Can you work these out from the model? Positions are in its coordinate system, mm. Face numbers are marked on the shaded views. A direction names the side the tool comes from. Give positions to 0.01 mm unless a question says otherwise; leave off trailing zeros. Write each loop counter-clockwise with the first axis right and the second up, starting at its lowest first coordinate (ties: lowest second). Pieces come first, ordered by that corner, then holes.
1. Suppose I cut it at A-A (y = 28). Please give me the cut outline in (x, z) (1 decimal).
2. Suppose I cut it at B-B (y = 21). Please give me the cut outline in (x, z) (3 decimals), and give its area (3 significant figures).
3. On a 3-axis mill with a long thin cutter (end or side, diameter ignored), from which of +Z, -Z, +X, -X, +Y, -Y can I reach the whole of each face in a straight line? I mean the marked faces 1 and 2. Say none if no direction works.
4. I'm going to push flat-ended pins straight in: pin 1 (2.5 mm diameter, centred on x = 74.61, z = 4.76, fed in from -Y); pin 2 (3 mm diameter, centred on x = 4.76, z = 74.61, fed in from +Y); pin 3 (2.5 mm diameter, centred on x = 4.76, z = 74.61, fed in from +Y). Where does each tip first touch, or does it pass through?
5. Suppose I cut it at C-C (x = 56). Please give me the cut outline in (y, z) (3 decimals).
6. If I drill on probe 1 along X at (y, z) = (20.5, 93) (3 decimals); probe 2 along Z at (x, y) = (75, 6) (3 decimals), over which ranges is the centre line in solid material (lowest first)?
7. Suppose I cut it at D-D (z = 98.5). Please give me the cut outline in (x, y) (3 decimals).
```python
from build123d import *

# Parameters (mm, degrees)
BOSS_EXTRUDE1_DEPTH                           = 38.1
CBORE_FOR_4_SOCKET_HEAD_CAP_SCREW1_AT_2_COUNT = 2
CBORE_FOR_4_SOCKET_HEAD_CAP_SCREW1_AT_2_PITCH = 34.925
CBORE_FOR_4_SOCKET_HEAD_CAP_SCREW1_AT_3_COUNT = 2
CBORE_FOR_4_SOCKET_HEAD_CAP_SCREW1_AT_3_PITCH = 69.85
CBORE_FOR_4_SOCKET_HEAD_CAP_SCREW1_AT_4_COUNT = 2
CBORE_FOR_4_SOCKET_HEAD_CAP_SCREW1_AT_4_PITCH = 34.925
CBORE_FOR_4_SOCKET_HEAD_CAP_SCREW1_AT_5_COUNT = 2
CBORE_FOR_4_SOCKET_HEAD_CAP_SCREW1_AT_5_PITCH = 69.85
CBORE_FOR_4_SOCKET_HEAD_CAP_SCREW1_AT_6_COUNT = 2
CBORE_FOR_4_SOCKET_HEAD_CAP_SCREW1_AT_6_PITCH = 104.775
CHAMFER1_SIZE                                 = 0.508


with BuildPart() as part:
    # Sketch1 → Boss-Extrude1 (new body)
    with BuildSketch(Plane(origin=(0, 0, 0), x_dir=(1, 0, 0), z_dir=(0, 1, 0))):
        Polygon((0, 0), (85.725, 0), (85.725, -9.525), (9.525, -9.525), (9.525, -123.825), (0, -123.825), align=None)
    extrude(amount=BOSS_EXTRUDE1_DEPTH)

    # Sketch2 → CBORE for #4 Socket Head Cap Screw1 (revolve, cut)
    with BuildSketch(Plane(origin=(4.7625, 0, 4.7625), x_dir=(0, 0, -1), z_dir=(1, 0, 0))):
        Polygon((0, 0), (0, 13.680574487), (1.63195, 12.7), (1.63195, 4.7625), (1.984375, 4.7625), (1.984375, 0), align=None)
    cbore_for_4_socket_head_cap_screw1 = revolve(axis=Axis((4.7625, -6.35, 4.7625), (0, 1, 0)), mode=Mode.SUBTRACT)

    # CBORE for #4 Socket Head Cap Screw1 at 2: CBORE for #4 Socket Head Cap Screw1 ×2
    with Locations(*[(0, 0, i * CBORE_FOR_4_SOCKET_HEAD_CAP_SCREW1_AT_2_PITCH) for i in range(1, CBORE_FOR_4_SOCKET_HEAD_CAP_SCREW1_AT_2_COUNT)]):
        add(cbore_for_4_socket_head_cap_screw1, mode=Mode.SUBTRACT)

    # CBORE for #4 Socket Head Cap Screw1 at 3: CBORE for #4 Socket Head Cap Screw1 ×2
    with Locations(*[(0, 0, i * CBORE_FOR_4_SOCKET_HEAD_CAP_SCREW1_AT_3_PITCH) for i in range(1, CBORE_FOR_4_SOCKET_HEAD_CAP_SCREW1_AT_3_COUNT)]):
        add(cbore_for_4_socket_head_cap_screw1, mode=Mode.SUBTRACT)

    # CBORE for #4 Socket Head Cap Screw1 at 4: CBORE for #4 Socket Head Cap Screw1 ×2
    with Locations(*[(i * CBORE_FOR_4_SOCKET_HEAD_CAP_SCREW1_AT_4_PITCH, 0, 0) for i in range(1, CBORE_FOR_4_SOCKET_HEAD_CAP_SCREW1_AT_4_COUNT)]):
        add(cbore_for_4_socket_head_cap_screw1, mode=Mode.SUBTRACT)

    # CBORE for #4 Socket Head Cap Screw1 at 5: CBORE for #4 Socket Head Cap Screw1 ×2
    with Locations(*[(i * CBORE_FOR_4_SOCKET_HEAD_CAP_SCREW1_AT_5_PITCH, 0, 0) for i in range(1, CBORE_FOR_4_SOCKET_HEAD_CAP_SCREW1_AT_5_COUNT)]):
        add(cbore_for_4_socket_head_cap_screw1, mode=Mode.SUBTRACT)

    # CBORE for #4 Socket Head Cap Screw1 at 6: CBORE for #4 Socket Head Cap Screw1 ×2
    with Locations(*[(0, 0, i * CBORE_FOR_4_SOCKET_HEAD_CAP_SCREW1_AT_6_PITCH) for i in range(1, CBORE_FOR_4_SOCKET_HEAD_CAP_SCREW1_AT_6_COUNT)]):
        add(cbore_for_4_socket_head_cap_screw1, mode=Mode.SUBTRACT)

    # Mirror CBORE for #4 Socket Head Cap Screw: CBORE for #4 Socket Head Cap Screw1 across plane
    add(cbore_for_4_socket_head_cap_screw1.mirror(Plane.ZX.offset(19.05)), mode=Mode.SUBTRACT)

    # Mirror CBORE for _4 Socket Head Cap  2 → Mirror CBORE for _4 Socket Head Cap  3 (revolve, cut)
    with BuildSketch(Plane(origin=(4.7625, 38.1, 39.6875), x_dir=(0, 0, -1), z_dir=(1, 0, 0))):
        Polygon((0, 0), (0, -13.680574487), (1.63195, -12.7), (1.63195, -4.7625), (1.984375, -4.7625), (1.984375, 0), align=None)
    revolve(axis=Axis((4.7625, 44.45, 39.6875), (0, 1, 0)), mode=Mode.SUBTRACT)

    # Mirror CBORE for _4 Socket Head Cap  4 → Mirror CBORE for _4 Socket Head Cap  5 (revolve, cut)
    with BuildSketch(Plane(origin=(4.7625, 38.1, 74.6125), x_dir=(0, 0, -1), z_dir=(1, 0, 0))):
        Polygon((0, 0), (0, -13.680574487), (1.63195, -12.7), (1.63195, -4.7625), (1.984375, -4.7625), (1.984375, 0), align=None)
    revolve(axis=Axis((4.7625, 44.45, 74.6125), (0, 1, 0)), mode=Mode.SUBTRACT)

    # Mirror CBORE for _4 Socket Head Cap  6 → Mirror CBORE for _4 Socket Head Cap  7 (revolve, cut)
    with BuildSketch(Plane(origin=(39.6875, 38.1, 4.7625), x_dir=(0, 0, -1), z_dir=(1, 0, 0))):
        Polygon((0, 0), (0, -13.680574487), (1.63195, -12.7), (1.63195, -4.7625), (1.984375, -4.7625), (1.984375, 0), align=None)
    revolve(axis=Axis((39.6875, 44.45, 4.7625), (0, 1, 0)), mode=Mode.SUBTRACT)

    # Mirror CBORE for _4 Socket Head Cap  8 → Mirror CBORE for _4 Socket Head Cap  9 (revolve, cut)
    with BuildSketch(Plane(origin=(74.6125, 38.1, 4.7625), x_dir=(0, 0, -1), z_dir=(1, 0, 0))):
        Polygon((0, 0), (0, -13.680574487), (1.63195, -12.7), (1.63195, -4.7625), (1.984375, -4.7625), (1.984375, 0), align=None)
    revolve(axis=Axis((74.6125, 44.45, 4.7625), (0, 1, 0)), mode=Mode.SUBTRACT)

    # Mirror CBORE for _4 Socket Head Cap  10 → Mirror CBORE for _4 Socket Head Cap  11 (revolve, cut)
    with BuildSketch(Plane(origin=(4.7625, 38.1, 109.5375), x_dir=(0, 0, -1), z_dir=(1, 0, 0))):
        Polygon((0, 0), (0, -13.680574487), (1.63195, -12.7), (1.63195, -4.7625), (1.984375, -4.7625), (1.984375, 0), align=None)
    revolve(axis=Axis((4.7625, 44.45, 109.5375), (0, 1, 0)), mode=Mode.SUBTRACT)

    # Chamfer1
    # the kernel refuses this chamfer: 0.508 mm, written as the material it adds along each edge
    with BuildSketch(Plane(origin=(4.7625, 4.7625, 4.7625), x_dir=(0, 0, -1), z_dir=(1, 0, 0))) as chamfer1_piece_1_section:
        Polygon((1.984375, -CHAMFER1_SIZE), (1.984375 - CHAMFER1_SIZE, 0), (1.984375, 0), align=None)
    chamfer1_piece_1 = revolve(axis=Axis((4.7625, 4.7625, 4.7625), (0, 1, 0)), mode=Mode.PRIVATE)
    chamfer1_piece_1 = chamfer1_piece_1 - Plane(origin=(4.7625, 4.431570678, 4.7625), x_dir=(0, 0, -1), z_dir=(0, -1, 0)) * Cylinder(1.63195, 8, mode=Mode.PRIVATE)
    add(chamfer1_piece_1)
    with BuildSketch(Plane(origin=(4.7625, 4.7625, 74.6125), x_dir=(0, 0, -1), z_dir=(1, 0, 0))) as chamfer1_piece_2_section:
        Polygon((1.984375, -CHAMFER1_SIZE), (1.984375 - CHAMFER1_SIZE, 0), (1.984375, 0), align=None)
    chamfer1_piece_2 = revolve(axis=Axis((4.7625, 4.7625, 74.6125), (0, 1, 0)), mode=Mode.PRIVATE)
    chamfer1_piece_2 = chamfer1_piece_2 - Plane(origin=(4.7625, 4.431570678, 74.6125), x_dir=(0, 0, -1), z_dir=(0, -1, 0)) * Cylinder(1.63195, 8, mode=Mode.PRIVATE)
    add(chamfer1_piece_2)
    with BuildSketch(Plane(origin=(39.6875, 33.3375, 4.7625), x_dir=(0, 0, -1), z_dir=(1, 0, 0))) as chamfer1_piece_3_section:
        Polygon((1.984375, CHAMFER1_SIZE), (1.984375 - CHAMFER1_SIZE, 0), (1.984375, 0), align=None)
    chamfer1_piece_3 = revolve(axis=Axis((39.6875, 33.3375, 4.7625), (0, 1, 0)), mode=Mode.PRIVATE)
    chamfer1_piece_3 = chamfer1_piece_3 - Plane(origin=(39.6875, 33.668429322, 4.7625), x_dir=(0, 0, -1), z_dir=(0, 1, 0)) * Cylinder(1.63195, 8, mode=Mode.PRIVATE)
    add(chamfer1_piece_3)
    # the kernel refuses this chamfer: 0.508 mm, written as the material it takes off along each edge
    with BuildSketch(Plane(origin=(4.7625, 0, 4.7625), x_dir=(0, 0, -1), z_dir=(1, 0, 0))) as chamfer1_2_piece_1:
        Polygon((1.984375 + CHAMFER1_SIZE, 0), (1.984375, CHAMFER1_SIZE), (1.984375, 0), align=None)
    revolve(axis=Axis((4.7625, 0, 4.7625), (0, 1, 0)), mode=Mode.SUBTRACT)
    with BuildSketch(Plane(origin=(4.7625, 0, 74.6125), x_dir=(0, 0, -1), z_dir=(1, 0, 0))) as chamfer1_2_piece_2:
        Polygon((1.984375 + CHAMFER1_SIZE, 0), (1.984375, CHAMFER1_SIZE), (1.984375, 0), align=None)
    revolve(axis=Axis((4.7625, 0, 74.6125), (0, 1, 0)), mode=Mode.SUBTRACT)
    with BuildSketch(Plane(origin=(74.6125, 0, 4.7625), x_dir=(0, 0, -1), z_dir=(1, 0, 0))) as chamfer1_2_piece_3:
        Polygon((1.984375 + CHAMFER1_SIZE, 0), (1.984375, CHAMFER1_SIZE), (1.984375, 0), align=None)
    revolve(axis=Axis((74.6125, 0, 4.7625), (0, 1, 0)), mode=Mode.SUBTRACT)
    with BuildSketch(Plane(origin=(39.6875, 0, 4.7625), x_dir=(0, 0, -1), z_dir=(1, 0, 0))) as chamfer1_2_piece_4:
        Polygon((1.984375 + CHAMFER1_SIZE, 0), (1.984375, CHAMFER1_SIZE), (1.984375, 0), align=None)
    revolve(axis=Axis((39.6875, 0, 4.7625), (0, 1, 0)), mode=Mode.SUBTRACT)
    with BuildSketch(Plane(origin=(4.7625, 0, 39.6875), x_dir=(0, 0, -1), z_dir=(1, 0, 0))) as chamfer1_2_piece_5:
        Polygon((1.984375 + CHAMFER1_SIZE, 0), (1.984375, CHAMFER1_SIZE), (1.984375, 0), align=None)
    revolve(axis=Axis((4.7625, 0, 39.6875), (0, 1, 0)), mode=Mode.SUBTRACT)
    with BuildSketch(Plane(origin=(4.7625, 0, 109.5375), x_dir=(0, 0, -1), z_dir=(1, 0, 0))) as chamfer1_2_piece_6:
        Polygon((1.984375 + CHAMFER1_SIZE, 0), (1.984375, CHAMFER1_SIZE), (1.984375, 0), align=None)
    revolve(axis=Axis((4.7625, 0, 109.5375), (0, 1, 0)), mode=Mode.SUBTRACT)
    with BuildSketch(Plane(origin=(39.6875, 38.1, 4.7625), x_dir=(0, 0, -1), z_dir=(1, 0, 0))) as chamfer1_2_piece_7:
        Polygon((1.984375 + CHAMFER1_SIZE, 0), (1.984375, -CHAMFER1_SIZE), (1.984375, 0), align=None)
    revolve(axis=Axis((39.6875, 38.1, 4.7625), (0, 1, 0)), mode=Mode.SUBTRACT)
    with BuildSketch(Plane(origin=(74.6125, 38.1, 4.7625), x_dir=(0, 0, -1), z_dir=(1, 0, 0))) as chamfer1_2_piece_8:
        Polygon((1.984375 + CHAMFER1_SIZE, 0), (1.984375, -CHAMFER1_SIZE), (1.984375, 0), align=None)
    revolve(axis=Axis((74.6125, 38.1, 4.7625), (0, 1, 0)), mode=Mode.SUBTRACT)
    with BuildSketch(Plane(origin=(4.7625, 38.1, 4.7625), x_dir=(0, 0, -1), z_dir=(1, 0, 0))) as chamfer1_2_piece_9:
        Polygon((1.984375 + CHAMFER1_SIZE, 0), (1.984375, -CHAMFER1_SIZE), (1.984375, 0), align=None)
    revolve(axis=Axis((4.7625, 38.1, 4.7625), (0, 1, 0)), mode=Mode.SUBTRACT)
    with BuildSketch(Plane(origin=(4.7625, 38.1, 39.6875), x_dir=(0, 0, -1), z_dir=(1, 0, 0))) as chamfer1_2_piece_10:
        Polygon((1.984375 + CHAMFER1_SIZE, 0), (1.984375, -CHAMFER1_SIZE), (1.984375, 0), align=None)
    revolve(axis=Axis((4.7625, 38.1, 39.6875), (0, 1, 0)), mode=Mode.SUBTRACT)
    with BuildSketch(Plane(origin=(4.7625, 38.1, 74.6125), x_dir=(0, 0, -1), z_dir=(1, 0, 0))) as chamfer1_2_piece_11:
        Polygon((1.984375 + CHAMFER1_SIZE, 0), (1.984375, -CHAMFER1_SIZE), (1.984375, 0), align=None)
    revolve(axis=Axis((4.7625, 38.1, 74.6125), (0, 1, 0)), mode=Mode.SUBTRACT)
    with BuildSketch(Plane(origin=(4.7625, 38.1, 109.5375), x_dir=(0, 0, -1), z_dir=(1, 0, 0))) as chamfer1_2_piece_12:
        Polygon((1.984375 + CHAMFER1_SIZE, 0), (1.984375, -CHAMFER1_SIZE), (1.984375, 0), align=None)
    revolve(axis=Axis((4.7625, 38.1, 109.5375), (0, 1, 0)), mode=Mode.SUBTRACT)


solid = part.part
```
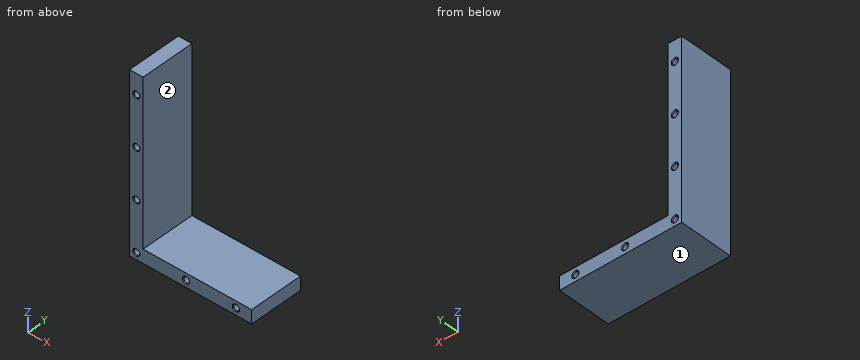
Checks:
1. outline: (0, 0) - (85.7, 0) - (85.7, 9.5) - (9.5, 9.5) - (9.5, 123.8) - (0, 123.8) - close; hole circle Ø3.3 at (4.8, 4.8); hole circle Ø3.3 at (4.8, 39.7); hole circle Ø3.3 at (4.8, 74.6); hole circle Ø3.3 at (4.8, 109.5); hole circle Ø3.3 at (39.7, 4.8); hole circle Ø3.3 at (74.6, 4.8)
2. outline: (0, 0) - (85.725, 0) - (85.725, 9.525) - (9.525, 9.525) - (9.525, 123.825) - (0, 123.825) - close
2. area: 1,910 mm2
3. face 1: -Z, +X, -X, +Y, -Y
3. face 2: +Z, +X, +Y, -Y
4. pin 1: stops at y = 12.93
4. pin 2: stops at y = 25.32
4. pin 3: stops at y = 25.17
5. outline: (0, 0) - (38.1, 0) - (38.1, 9.525) - (0, 9.525) - close
6. probe 1: x = 0 to 9.525
6. probe 2: z = 0 to 3.177, 6.348 to 9.525
7. outline: (0, 0) - (9.525, 0) - (9.525, 38.1) - (0, 38.1) - close
